Input: dimensioned drawing with shaded views. Units: mm. Origin: part minimum x, y, z. A direction names the side the tool comes from. Give positions to 0.01 mm unless a question says otherwise; leave off trailing zeros. Write each loop counter-clockwise with the first axis right and the second up, starting at its lowest first coordinate (ties: lowest second). Pieces come first, ordered by that corner, then holes. Notation, with made-up numbers: (-25, -5) -> (29, -5) arc R12 cw to (29, 11) -> close; hole circle Ø11 at (44.5, 88). An arc over 180 degrees is marked (long way). Return JSON: item names as keys, results as strings. Group by question number.
Item 1: Section C-C, the plane x = 7. Return loops of the section in (y, z).
Item 2: Set-up query: the marked faces 5 and 6. Return all of +Z, -Z, +X, -X, +Y, -Y with unobstructed straight access to the full face (end or side cutting, diameter ignored); none if empty.
Item 3: Pin query (flat end, axial travel): P1, Ø2, axis at y = 3, z = 3, coming from the -X side; P2, Ø3, axis at x = 4, y = 1.5, coming from the -Z side; P3, Ø4, axis at y = 7, z = 5.5, coming from the +X side (1 decimal); P4, Ø1.5, axis at x = 9.5, z = 5, coming from the +Y side. Return the tip coordinate at first contact, or that it passes through.
Item 4: Section A-A, the plane x = 5. Return loops of the section in (y, z), then the cut area to 3 significant figures.
Item 5: Line query: line 1 (X direction, y = 5.25, z = 6.5); line 2 (X direction, y = 2.5, z = 4.25); line 3 (X direction, y = 5.75, z = 5.5). Output: solid intervals per line, ascending. Write a range as [from, to].
Item 6: Section B-B, the plane z = 1.5. Return loops of the section in (x, y) (1 decimal).
Item 7: Mould query, pull axis X, two halves, no side actions, for the marked faces 1, 2, 3 and 4. Classes: released by +X, released by -X, zero draft, split by the parting line, or undercut.
Item 8: Section D-D, the plane y = 7.75. Return loops of the section in (x, z).
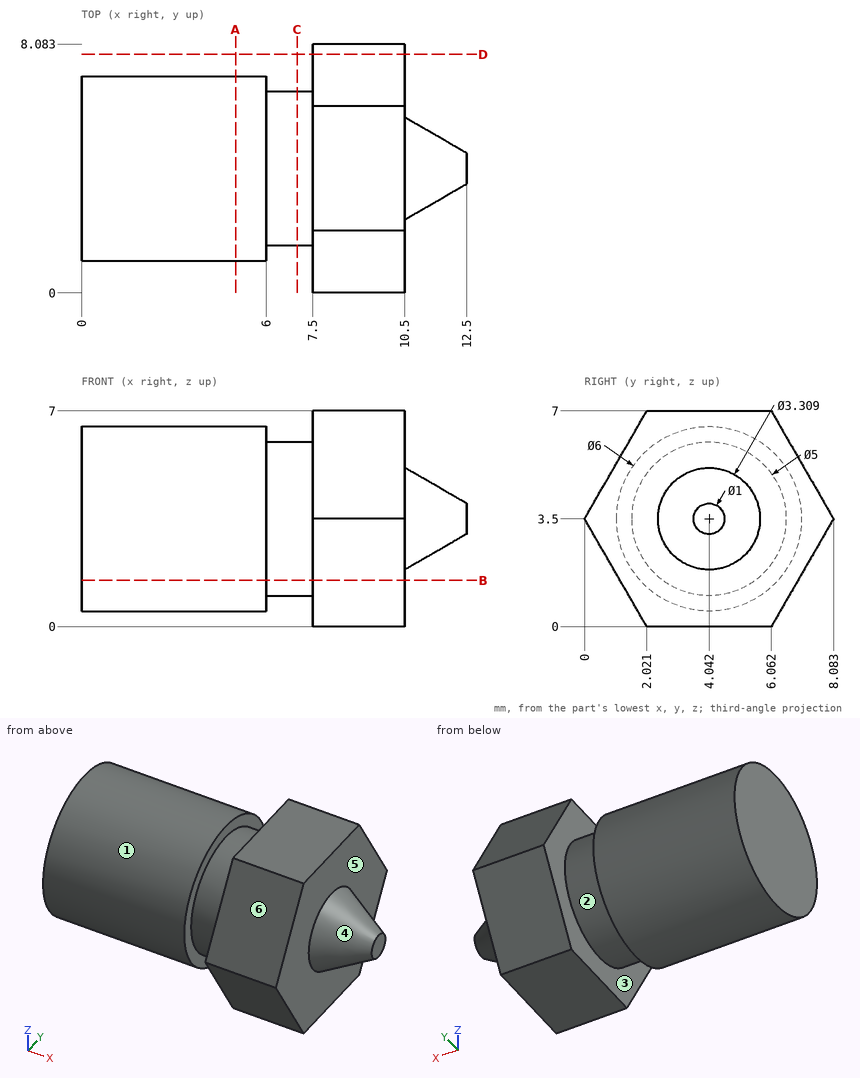
Answer below:
{
 "1": {"outline": "circle Ø5 at (4.04, 3.5)"},
 "2": {"face 5": "+X", "face 6": "+Z, +X, -X, -Y"},
 "3": {"P1": "stops at x = 0", "P2": "stops at z = 0.69", "P3": "stops at x = 10.6", "P4": "stops at y = 7.65"},
 "4": {"outline": "circle Ø6 at (4.04, 3.5)", "area": "28.3 mm2"},
 "5": {"line 1": "x = [7.5, 10.5]", "line 2": "x = [0, 10.5]", "line 3": "x = [0, 6], [7.5, 10.5]"},
 "6": {"outline": "(0, 1.8) -> (6, 1.8) -> (6, 2.5) -> (7.5, 2.5) -> (7.5, 1.2) -> (10.5, 1.2) -> (10.5, 6.9) -> (7.5, 6.9) -> (7.5, 5.5) -> (6, 5.5) -> (6, 6.3) -> (0, 6.3) -> close"},
 "7": {"face 1": "zero draft", "face 2": "undercut", "face 3": "undercut", "face 4": "released by +X"},
 "8": {"outline": "(7.5, 2.92) -> (10.5, 2.92) -> (10.5, 4.08) -> (7.5, 4.08) -> close"}
}
